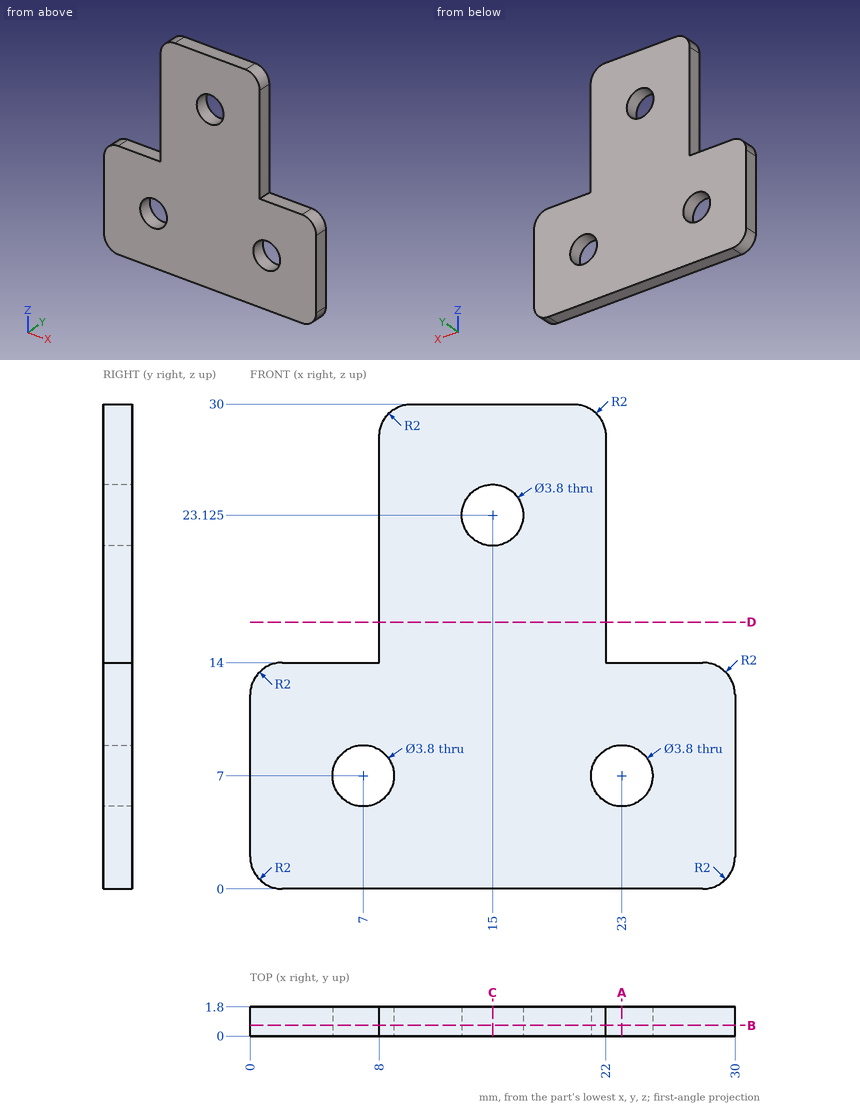
Print and shaded views of the part. All mm, measured from the part's lowest x, y and z. Give positions to 0.01 mm unless a question says otherwise; leave off trailing zeros. Loops run counter-clockwise (first coordinate to the right, second up) from the corner with the lowest first, then second, coordinate; pieces in that order, holes last. Notation, with made-up numbers: (-33, 13) -> (23, 13) arc R21 ccw to (23, 18) -> close; hole circle Ø4 at (-7, 76). An arc over 180 degrees is marked (long way). Use CSV: the item, a comma, the result in double quotes. Start each with the question number.
1) Slice it at D-D on z = 16.5. Give the cut face in (x, y), plus the area to 3 significant figures.
2) Flat gauge pins, fed straight in: pin 1 Ø0.9 at (x, y) = (25.5, 0.5) entering from +Z; pin 2 Ø0.9 at (y, z) = (1, 19) entering from +X. Where does each tip first touch, or does it go through?
3) Wall check: line 1 (X direction, y = 1, z = 7); line 2 (X direction, y = 0.9, z = 8) (1 decimal); line 3 (X direction, y = 0.5, z = 20). Give the ranges that are in metal, low to high.
4) Slice it at A-A on x = 23. Give the cut face in (y, z).
5) Slice it at C-C on x = 15. Give the cut face in (y, z) (1 decimal).
6) Slice it at B-B on y = 0.65. Give the cut face in (x, z) (1 decimal).
Computed values:
1,outline,"(8, 0) -> (22, 0) -> (22, 1.8) -> (8, 1.8) -> close"
1,area,"25.2 mm^2"
2,pin 1,"stops at z = 14"
2,pin 2,"stops at x = 22"
3,line 1,"x = 0 to 5.1, 8.9 to 21.1, 24.9 to 30"
3,line 2,"x = 0 to 5.4, 8.6 to 21.4, 24.6 to 30"
3,line 3,"x = 8 to 22"
4,outline,"(0, 0) -> (1.8, 0) -> (1.8, 5.1) -> (0, 5.1) -> close; (0, 8.9) -> (1.8, 8.9) -> (1.8, 14) -> (0, 14) -> close"
5,outline,"(0, 0) -> (1.8, 0) -> (1.8, 21.2) -> (0, 21.2) -> close; (0, 25) -> (1.8, 25) -> (1.8, 30) -> (0, 30) -> close"
6,outline,"(0, 2) arc R2 ccw to (2, 0) -> (28, 0) arc R2 ccw to (30, 2) -> (30, 12) arc R2 ccw to (28, 14) -> (22, 14) -> (22, 28) arc R2 ccw to (20, 30) -> (10, 30) arc R2 ccw to (8, 28) -> (8, 14) -> (2, 14) arc R2 ccw to (0, 12) -> close; hole circle Ø3.8 at (7, 7); hole circle Ø3.8 at (15, 23.1); hole circle Ø3.8 at (23, 7)"
